For this review, take the finished solid that the model builds, in its own axes (mm). A direction names the side the tool comes from. Coordinates: 2 decimals unless noted, no trailing zeros. Order: outer loops, then holes, each group sorted by start corner. A loop starts at its lowest first (then second) coordinate and runs counter-clockwise, first axis right, second up. Notation, with made-up numbers: (-6, -36) -> (51, -36) arc R25 ccw to (51, -7) -> close; hole circle Ø10 at (87.25, 78). An arc over 180 degrees is marked (long way). Answer as a JSON object with one key per item and string values. Group by question number.
1) Add section B-B, the plane x = -17.5. Write out the cut boundary in (y, z) (3 decimals), then the cut area to 3 significant figures.
2) For pin 1 (1 mm diameter, centred on x = 10, z = 2, fed in from +Y); pin 2 (1.5 mm diameter, centred on y = -21, z = 4.5, fed in from +X); pin 3 (3 mm diameter, centred on y = -19.5, z = 2, fed in from +X); pin 4 (5 mm diameter, centred on x = -14.5, y = -7.5, fed in from -Z), all flat-tipped, find the tip position at first contact; note any pin that passes through.
3) Add section A-A, the plane y = 0. Write out the cut boundary in (x, z) (1 decimal).
4) Add section D-D, the plane x = 21. Write out the cut boundary in (y, z) (3 decimals), then the cut area to 3 significant figures.
5) Machinability: for faces 5 (the flat face through (-11, -5, 0)), 6 (the flat face through (-18.6, -20, 3)), which of the approach directions +Z, -Z, +X, -X, +Y, -Y give a long, thin tool a straight path to every point of the face, cutting with its end or side? Answer none if there is none.
6) Add section C-C, the plane z = 5.25. Count the separate pieces of the cut face and the enclosed holes in it, then the cut area to 3 significant figures.
7) Wall thickness on L1, parallel to Y at x = -16.5, z = 4.5; L2, parallel to Y at x = -12, z = 5; L3, parallel to Y at x = 15, z = 3: over which ranges is each line inside the solid? List them lowest first.
8) Draft analysis for pull direction X (two halves, no side actions). For faces 1 (the flat face through (-11, -5, 6.985)), 2 (the flat face through (26.48, 6.19, 3.44)), 3 (the flat face through (-22.41, -20, 3)), 4 (the flat face through (33.898, 0, 3)), state which applies: +X half, -X half, draft (parallel to the pull), parting line (faces both ways), or undercut.
from build123d import *

# Parameters (mm, degrees)
F0_R     = 10.9855
F1_DEPTH = 6.985


with BuildPart() as f1:
    # F0 (on Top) → F1 (new body)
    with BuildSketch(Plane.XY):
        with BuildLine():
            Line((-0.570141, 26.199883), (-0.570143, 26.205813))
            Line((-0.570143, 26.205813), (-11.487829, 32.509142))
            Line((-11.487829, 32.509142), (-22.409829, 26.203322))
            Line((-22.409829, 26.203322), (-22.409829, 13.591683))
            ThreePointArc((-22.409829, 13.591683), (-14.562667, 0), (-22.409828, -13.591683))
            Line((-22.409828, -13.591683), (-22.409828, -26.203322))
            Line((-22.409828, -26.203322), (-11.487828, -32.509142))
            Line((-11.487828, -32.509142), (-0.565829, -26.203322))
            ThreePointArc((-0.565829, -26.203322), (7.280049, -12.609415), (22.975657, -12.608674))
            Line((22.975657, -12.608674), (33.897656, -6.302854))
            Line((33.897656, -6.302854), (33.897656, 6.308785))
            Line((33.897656, 6.308785), (22.975657, 12.614604))
            ThreePointArc((22.975657, 12.614604), (7.282309, 12.612381), (-0.570141, 26.199883))
        make_face()
        Polygon((-18.599828, -24.003618), (-18.599828, -15.791388), (-11.487828, -11.685272), (-4.375828, -15.791388), (-4.375828, -24.003618), (-11.487828, -28.109733), align=None, mode=Mode.SUBTRACT)
        Circle(F0_R, mode=Mode.SUBTRACT)
        Polygon((22.975657, -8.21223), (15.863657, -4.106115), (15.863657, 4.106115), (22.975657, 8.21223), (30.087657, 4.106115), (30.087657, -4.106115), align=None, mode=Mode.SUBTRACT)
        Polygon((-11.487829, 28.109733), (-4.375829, 24.003618), (-4.375829, 15.791387), (-11.487829, 11.685272), (-18.599829, 15.791387), (-18.599829, 24.003618), align=None, mode=Mode.SUBTRACT)
    extrude(amount=F1_DEPTH)


solid = f1.part
Output values:
{
 "1": {"outline": "(-29.038, 0) -> (-24.639, 0) -> (-24.639, 6.985) -> (-29.038, 6.985) -> close; (-15.156, 0) -> (-9.142, 0) -> (-9.142, 6.985) -> (-15.156, 6.985) -> close; (9.142, 0) -> (15.156, 0) -> (15.156, 6.985) -> (9.142, 6.985) -> close; (24.639, 0) -> (29.038, 0) -> (29.038, 6.985) -> (24.639, 6.985) -> close", "area": "145 mm²"},
 "2": {"pin 1": "stops at y = 11.55", "pin 2": "stops at x = 0.61", "pin 3": "stops at x = 1.75", "pin 4": "stops at z = 0"},
 "3": {"outline": "(-14.6, 0) -> (-11, 0) -> (-11, 7) -> (-14.6, 7) -> close; (11, 0) -> (15.9, 0) -> (15.9, 7) -> (11, 7) -> close; (30.1, 0) -> (33.9, 0) -> (33.9, 7) -> (30.1, 7) -> close"},
 "4": {"outline": "(-11.646, 0) -> (-7.072, 0) -> (-7.072, 6.985) -> (-11.646, 6.985) -> close; (7.072, 0) -> (11.652, 0) -> (11.652, 6.985) -> (7.072, 6.985) -> close", "area": "63.9 mm²"},
 "5": {"face 5": "-Z, +X, -X, +Y, -Y", "face 6": "+Z, -Z"},
 "6": {"separate pieces": "1", "enclosed holes": "4", "area": "1,040 mm²"},
 "7": {"L1": "y = -29.62 to -25.22, -14.58 to -7.55, 7.55 to 14.58, 25.22 to 29.62", "L2": "y = -32.21 to -27.81, -11.98 to 11.98, 27.81 to 32.21", "L3": "y = -10.51 to 10.51"},
 "8": {"face 1": "draft", "face 2": "undercut", "face 3": "-X half", "face 4": "+X half"}
}
